The model under review builds one solid part; all positions refer to its coordinate system, in mm. A direction names the side the tool comes from. Give positions to 0.01 mm unless a question says otherwise; leave off trailing zeros. Loops run counter-clockwise (first coordinate to the right, second up) from the corner with the lowest first, then second, coordinate; pieces in that order, holes last. Notation, with made-up numbers: M -32.5,81 L 17.5,81 A13 cw 17.5,93 Z; hole C 7,13.25 d10. An arc over 180 degrees is marked long. One line per item, written item: value. Start each with the question number.
Q1. We need section A-A on y = -47. Write out the cut boundary in (x, z) (3 decimals).
Q2. For faces 1 (the face through (2.4, 0, 2.4)), 2 (the face through (0, 2, -5.556)), list the 3-axis set-ups (+Z, -Z, +X, -X, +Y, -Y) from which the entire face can be reached by the end or side of a thin tool; tool diameter is ignored.
Q3. For pin 1 (1.3 mm diameter, centred on x = -5, z = 0.5, fed in from -Y); pin 2 (5 mm diameter, centred on y = -39, z = 3.5, fed in from +X); pin 3 (4 mm diameter, centred on x = -1.5, y = -178.5, fed in from -Z) (3 decimals), all flat-tipped, find the tip position at first contact; note any pin that passes through.
Q4. To check wall thickness, follow line 1 along X through (y, z) = (-151, -1.5); line 2 along Z through (x, y) = (0.25, -109.5); line 3 along Y through (x, z) = (4.25, -2). State the ranges of each line that lie inside material, in increasing order. Write a range as from..to.
```python
from build123d import *

# Parameters (mm, degrees)
BASE_EXTRUDE_DEPTH  = 3.96875
SKETCH5_R           = 3.175
BOSS_EXTRUDE1_DEPTH = 203.2
CHAMFER1_SIZE       = 0.635
CHAMFER1_SIZE2      = 0.366617421


with BuildPart() as part:
    # Sketch4 → Base-Extrude (new body)
    with BuildSketch(Plane(origin=(0, 0, 0), x_dir=(1, 0, 0), z_dir=(0, 1, 0))):
        Polygon((6.415804866, 0), (3.207902433, 5.55625), (-3.207902433, 5.55625), (-6.415804866, 0), (-3.207902433, -5.55625), (3.207902433, -5.55625), align=None)
    extrude(amount=BASE_EXTRUDE_DEPTH)

    # Sketch5 → Boss-Extrude1 (add)
    with BuildSketch(Plane.XZ):
        with Locations(Location((0, 0, 0), (0, 0, 90))):
            Circle(SKETCH5_R)
    extrude(amount=BOSS_EXTRUDE1_DEPTH)

    # Sketch8 → Cut-Revolve1 (revolve, cut)
    with BuildSketch(Plane(origin=(0, 0, 0), x_dir=(0, 0, -1), z_dir=(1, 0, 0)), mode=Mode.PRIVATE) as cut_revolve1_sk:
        Polygon((5.55625, 3.96875), (11.726421194, 0.4064), (5.55625, 0.4064), (5.55625, 0), (14.266421194, 0), (14.266421194, 3.96875), align=None)
    revolve(cut_revolve1_sk.sketch.rotate(Axis((0, 0, 0), (0, 1, 0)), 180), axis=Axis((0, 0, 0), (0, 1, 0)), mode=Mode.SUBTRACT)

    # Chamfer1
    chamfer1_edges = [part.edges().sort_by_distance(p)[0] for p in [
        (0, -203.2, -3.175),
    ]]
    chamfer1_side = [part.faces().sort_by_distance(p)[0] for p in [
        (0, -203.2, 0),
    ]]
    chamfer(chamfer1_edges, length=CHAMFER1_SIZE, length2=CHAMFER1_SIZE2, reference=chamfer1_side[0])


solid = part.part
```
Solved:
1. outline: C 0,0 d6.35
2. face 1: -Y
2. face 2: -Z, +X, -X, +Y, -Y
3. pin 1: y = 0
3. pin 2: x = 3.01
3. pin 3: z = -3.175
4. line 1: -2.8..2.8
4. line 2: -3.17..3.17
4. line 3: 0..3.97
